```python
from build123d import *

# Parameters (mm, degrees)
SKETCH1_W           = 147.6375
SKETCH1_H           = 25.4
BOSS_EXTRUDE1_DEPTH = 3.175
SKETCH2_W           = 3.175
SKETCH2_H           = 25.4
BOSS_EXTRUDE2_DEPTH = 30.53588


with BuildPart() as part:
    # Sketch1 → Boss-Extrude1 (new body)
    with BuildSketch(Plane.XY):
        Rectangle(SKETCH1_W, SKETCH1_H)
    extrude(amount=BOSS_EXTRUDE1_DEPTH)

    # Sketch2 → Boss-Extrude2 (add)
    with BuildSketch(Plane.XY.offset(3.175)):
        with Locations((-72.23125, 0)):
            Rectangle(SKETCH2_W, SKETCH2_H)
    boss_extrude2 = extrude(amount=BOSS_EXTRUDE2_DEPTH)

    # Mirror1: Boss-Extrude2 across plane
    add(boss_extrude2.mirror(Plane(origin=(0, 0, 0), x_dir=(0, 0, 1), z_dir=(1, 0, 0))))


solid = part.part
```
Source: CAD feature listing. Evaluate the final solid. Frame: model axes, mm. A direction names the side the tool comes from. Give positions to 0.01 mm unless a question says otherwise; leave off trailing zeros. Write each loop counter-clockwise with the first axis right and the second up, starting at its lowest first coordinate (ties: lowest second). Pieces come first, ordered by that corner, then holes. Notation, with made-up numbers: (49.25, 41.5) - (76.25, 41.5) arc R20 cw to (76.25, 76.5) - close; hole circle Ø10 at (1, 27.25). An arc over 180 degrees is marked (long way). One line per item, written item: value. Start each with the question number.
Q1. Section query C-C, the plane x = -11.5. Return the cut outline in (y, z) (3 decimals), then the cut area to 3 significant figures.
Q2. Section query A-A, the plane z = 24. Return the cut outline in (x, y).
Q3. Draft query along X for faces 3 (the face through (-73.819, 0, 17)), 4 (the face through (-70.644, 0, 18)), 5 (the face through (-1, 0, 0)). Return one class per face: +X half, -X half, draft (parallel to the pull), parting line (faces both ways), or undercut.
Q4. Section query B-B, the plane y = -5.75. Return the cut outline in (x, z) (3 decimals).
Q5. Set-up query: faces 1 (the face through (72, 0, 33.711)), 2 (the face through (-1, 0, 3.175)). Return all of +Z, -Z, +X, -X, +Y, -Y with unobstructed straight access to the full face (end or side cutting, diameter ignored); none if empty.
Q6. Material intervals for probe 1 along X at (y, z) = (-8.75, 30.5); probe 2 along Z at (x, y) = (-49, 3.5) (3 decimals), sorted ascending. Write a range as from..to.
Q7. First-contact query: pin 1 Ø1.5 at (x, y) = (-23.5, 6.5) entering from +Z (3 decimals). Flat tip, straight axial feed; report the tip coordinate or a pass-through.
Answer:
1. outline: (-12.7, 0) - (12.7, 0) - (12.7, 3.175) - (-12.7, 3.175) - close
1. area: 80.6 mm2
2. outline: (-73.82, -12.7) - (-70.64, -12.7) - (-70.64, 12.7) - (-73.82, 12.7) - close; (70.64, -12.7) - (73.82, -12.7) - (73.82, 12.7) - (70.64, 12.7) - close
3. face 3: -X half
3. face 4: undercut
3. face 5: draft
4. outline: (-73.819, 0) - (73.819, 0) - (73.819, 33.711) - (70.644, 33.711) - (70.644, 3.175) - (-70.644, 3.175) - (-70.644, 33.711) - (-73.819, 33.711) - close
5. face 1: +Z, +X, -X, +Y, -Y
5. face 2: +Z, +Y, -Y
6. probe 1: x = -73.82..-70.64, 70.64..73.82
6. probe 2: z = 0..3.175
7. pin 1: stops at z = 3.175
